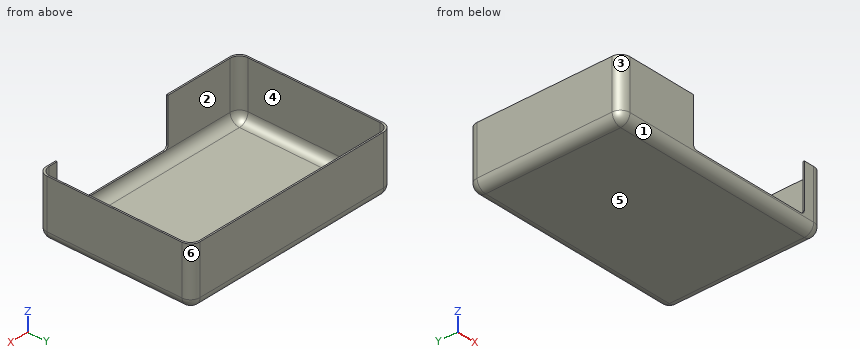
from build123d import *

# Parameters (mm, degrees)
BOSS_EXTRUDE1_DEPTH = 88.9
CUT_EXTRUDE1_DEPTH  = 86.614
FILLET1_R           = 14.224
FILLET2_R           = 14.224
CUT_EXTRUDE2_DEPTH  = 2.286


with BuildPart() as part:
    # Sketch1 → Boss-Extrude1 (new body)
    with BuildSketch(Plane.XY):
        with BuildLine():
            Line((-41.405944168, 22.056216238), (266.696055832, 22.056216238))
            ThreePointArc((266.696055832, 22.056216238), (276.753942688, 17.890103094), (280.920055832, 7.832216238))
            Line((280.920055832, 7.832216238), (280.920055832, -197.145783762))
            ThreePointArc((280.920055832, -197.145783762), (276.753942688, -207.203670617), (266.696055832, -211.369783762))
            Line((266.696055832, -211.369783762), (-41.405944168, -211.369783762))
            ThreePointArc((-41.405944168, -211.369783762), (-51.463831024, -207.203670617), (-55.629944168, -197.145783762))
            Line((-55.629944168, -197.145783762), (-55.629944168, 7.832216238))
            ThreePointArc((-55.629944168, 7.832216238), (-51.463831024, 17.890103094), (-41.405944168, 22.056216238))
        make_face()
    extrude(amount=BOSS_EXTRUDE1_DEPTH)

    # Sketch4 → Cut-Extrude1 (cut)
    with BuildSketch(Plane.XY.offset(88.9)):
        with BuildLine():
            Line((-39.119944168, -209.083783762), (264.410055832, -209.083783762))
            ThreePointArc((264.410055832, -209.083783762), (274.467942688, -204.917670617), (278.634055832, -194.859783762))
            Line((278.634055832, -194.859783762), (278.634055832, 5.546216238))
            ThreePointArc((278.634055832, 5.546216238), (274.467942688, 15.604103094), (264.410055832, 19.770216238))
            Line((264.410055832, 19.770216238), (-39.119944168, 19.770216238))
            ThreePointArc((-39.119944168, 19.770216238), (-49.177831024, 15.604103094), (-53.343944168, 5.546216238))
            Line((-53.343944168, 5.546216238), (-53.343944168, -194.859783762))
            ThreePointArc((-53.343944168, -194.859783762), (-49.177831024, -204.917670617), (-39.119944168, -209.083783762))
        make_face()
    extrude(amount=-CUT_EXTRUDE1_DEPTH, mode=Mode.SUBTRACT)

    # Fillet1
    fillet1_edges = [part.edges().sort_by_distance(p)[0] for p in [
        (-49.177831024, -204.917670617, 2.286),
        (-53.343944168, -94.656783762, 2.286),
        (-49.177831024, 15.604103094, 2.286),
        (112.645055832, 19.770216238, 2.286),
        (274.467942688, 15.604103094, 2.286),
        (278.634055832, -94.656783762, 2.286),
        (274.467942688, -204.917670617, 2.286),
        (112.645055832, -209.083783762, 2.286),
    ]]
    fillet(fillet1_edges, radius=FILLET1_R)

    # Fillet2
    fillet2_edges = [part.edges().sort_by_distance(p)[0] for p in [
        (-55.629944168, -94.656783762, 0),
        (-51.463831024, 17.890103094, 0),
        (112.645055832, 22.056216238, 0),
        (276.753942688, 17.890103094, 0),
        (280.920055832, -94.656783762, 0),
        (276.753942688, -207.203670617, 0),
        (112.645055832, -211.369783762, 0),
        (-51.463831024, -207.203670617, 0),
    ]]
    fillet(fillet2_edges, radius=FILLET2_R)

    # Sketch5 → Cut-Extrude2 (cut)
    with BuildSketch(Plane(origin=(0, -211.369783762, 0), x_dir=(-1, 0, 0), z_dir=(0, -1, 0))):
        with BuildLine():
            Line((-64.758151491, -88.9), (-64.758151491, -22.994419779))
            ThreePointArc((-64.758151491, -22.994419779), (-66.61802343, -18.504291719), (-71.108151491, -16.644419779))
            Line((-71.108151491, -16.644419779), (-244.615767903, -16.644419779))
            ThreePointArc((-244.615767903, -16.644419779), (-249.105895963, -18.504291719), (-250.965767903, -22.994419779))
            Line((-250.965767903, -22.994419779), (-250.965767903, -88.9))
            Line((-250.965767903, -88.9), (-64.758151491, -88.9))
        make_face()
    extrude(amount=-CUT_EXTRUDE2_DEPTH, mode=Mode.SUBTRACT)


solid = part.part
Build history of the part. All positions in model axes, mm. Face numbers are marked on the shaded views. A direction names the side the tool comes from. Round coordinates to 2 decimals unless told otherwise and drop trailing zeros. Write each loop counter-clockwise with the first axis right and the second up, starting at its lowest first coordinate (ties: lowest second). Pieces come first, ordered by that corner, then holes. Notation, with made-up numbers: M -13,73.5 L -3,73.5 A23 cw -3,93.5 Z; hole C 25.25,59 d9. An arc over 180 degrees is marked long. Answer as a JSON object with one key per item and string values. Group by question number.
(1) Cut at C-C (y = -185.5). Give the cut face in (x, z), and give its area (3 significant figures).
(2) Which spindle directions (+Z, -Z, +X, -X, +Y, -Y) get a long thin tool onto all of the face, cutting with end or side? Do the marked faces 1 and 2. Say none if no direction does.
(3) Cut at A-A (x = -8). Give the cut face in (y, z).
(4) Cut at B-B (z = 38). Give the cut face in (x, y).
(5) Mould opens along Y. For the marked faces 3, 4, 5 and 6 say: pulls with the +Y half, pulls with the -Y half, needs draft (parallel to the pull), parting line crosses it, or undercut.
(6) Flat gauge pins, fed straight in: pin 1 (1.1 mm diameter, centred on y = -210.5, z = 47, fed in from +X); pin 2 (1.8 mm diameter, centred on x = 178.5, y = -210.5, fed in from +Z); pin 3 (10 mm diameter, centred on x = 136.5, z = 64, fed in from -Y). Where does each tip first touch, or does it go through?
(7) Drill centre lines: L1, parallel to Y at x = 55, z = 68; L2, parallel to X at y = -35, z = 30; L3, parallel to Z at x = 80.5, y = -76. Where is each one in solid material? Low to high.
Responses:
{
 "1": {"outline": "M -55.63,14.22 A14.22 ccw -41.41,0 L 266.7,0 A14.22 ccw 280.92,14.22 L 280.92,88.9 L 278.63,88.9 L 278.63,16.51 A14.22 cw 264.41,2.29 L -39.12,2.29 A14.22 cw -53.34,16.51 L -53.34,88.9 L -55.63,88.9 Z", "area": "1,170 mm2"},
 "2": {"face 1": "-Z, +X, -X, -Y", "face 2": "+Z"},
 "3": {"outline": "M -211.37,14.22 A14.22 ccw -197.15,0 L 7.83,0 A14.22 ccw 22.06,14.22 L 22.06,88.9 L 19.77,88.9 L 19.77,16.51 A14.22 cw 5.55,2.29 L -194.86,2.29 A14.22 cw -209.08,16.51 L -209.08,88.9 L -211.37,88.9 Z"},
 "4": {"outline": "M -55.63,-197.15 A14.22 ccw -41.41,-211.37 L 64.76,-211.37 L 64.76,-209.08 L -39.12,-209.08 A14.22 cw -53.34,-194.86 L -53.34,5.55 A14.22 cw -39.12,19.77 L 264.41,19.77 A14.22 cw 278.63,5.55 L 278.63,-194.86 A14.22 cw 264.41,-209.08 L 250.97,-209.08 L 250.97,-211.37 L 266.7,-211.37 A14.22 ccw 280.92,-197.15 L 280.92,7.83 A14.22 ccw 266.7,22.06 L -41.41,22.06 A14.22 ccw -55.63,7.83 Z"},
 "5": {"face 3": "pulls with the -Y half", "face 4": "undercut", "face 5": "needs draft", "face 6": "pulls with the +Y half"},
 "6": {"pin 1": "stops at x = 272.89", "pin 2": "stops at z = 16.64", "pin 3": "stops at y = 19.77"},
 "7": {"L1": "y = -211.37 to -209.08, 19.77 to 22.06", "L2": "x = -55.63 to -53.34, 278.63 to 280.92", "L3": "z = 0 to 2.29"}
}
